```python
from build123d import *

# Parameters (mm, degrees)
SKETCH_R     = 9.65
PAD_DEPTH    = 100
FILLET_R     = 3
POCKET_DEPTH = 3


with BuildPart() as part:
    # Sketch → Pad (new body)
    with BuildSketch(Plane.XY):
        with BuildLine():
            ThreePointArc((0, 12.5), (-12.5, 0), (0, -12.5))
            Line((0, -12.5), (10.5, -12.5))
            Line((10.5, 12.5), (10.5, -12.5))
            Line((0, 12.5), (10.5, 12.5))
        make_face()
        Circle(SKETCH_R, mode=Mode.SUBTRACT)
    extrude(amount=PAD_DEPTH)

    # Fillet
    fillet_edges = [part.edges().sort_by_distance(p)[0] for p in [
        (10.5, -12.5, 50),
        (10.5, 12.5, 50),
    ]]
    fillet(fillet_edges, radius=FILLET_R)

    # Sketch001 (on DatumPlane) → Pocket (cut)
    with BuildSketch(Plane(origin=(-12.5, 0, 100), x_dir=(0, 0, -1), z_dir=(-1, 0, 0))):
        Polygon((12.979274, -3.5), (17.020726, -3.5), (19.041452, 0), (17.020726, 3.5), (12.979274, 3.5), (10.958548, 0), align=None)
        Polygon((87.020726, -3.5), (89.041452, 0), (87.020726, 3.5), (82.979274, 3.5), (80.958548, 0), (82.979274, -3.5), align=None)
    extrude(amount=-POCKET_DEPTH, mode=Mode.SUBTRACT)


solid = part.part
```
Input: part model. Units: mm. Frame: model coordinates. A direction names the side the tool comes from. Coordinates: 2 decimals unless noted, no trailing zeros. Write each loop counter-clockwise with the first axis right and the second up, starting at its lowest first coordinate (ties: lowest second). Pieces come first, ordered by that corner, then holes. Notation, with made-up numbers: (79.25, 16.25) -> (101.25, 16.25) arc R24 ccw to (101.25, 47.25) -> close; hole circle Ø7 at (6.25, 2). An arc over 180 degrees is marked (long way). Answer as a JSON object with one key per item and string values.
1. First-contact query: P1, Ø3, axis at x = -11.5, z = 85, coming from the -Y side; P2, Ø1.2, axis at x = -11.5, z = 15, coming from the +Y side; P3, Ø1, axis at y = 10, z = 29, coming from the -X side. Flat tips, straight axial feed; report the tip coordinate or a pass-through.
Result set:
{"P1": "stops at y = -7.5", "P2": "stops at y = 6.12", "P3": "stops at x = -8.12"}
2. Access query for faces 1 (the face through (-11, -3.5, 85)), 2 (the face through (-5.3, 8.4, 0)). Directions: +Z, -Z, +X, -X, +Y, -Y. A direction counts if a zero-diameter tool reaches every point of the face in a straight line with its end or side. Return the directions, or none.
Result set:
{"face 1": "-X", "face 2": "-Z, +X, -X, +Y, -Y"}
3. Mould query, pull axis Y, two halves, no side actions, for faces 3 (the face through (10.5, 0, 49)), 4 (the face through (-12.497, 0.275, 49.3)), 5 (the face through (-11, -3.5, 15)). Classes: released by +Y, released by -Y, zero draft, split by the parting line, or undercut.
Result set:
{"face 3": "zero draft", "face 4": "split by the parting line", "face 5": "undercut"}
4. Section B-B on x = -5.5. Return the cut outline in (y, z), then the cut area to 3 significant figures.
Result set:
{"outline": "(-11.22, 0) -> (-7.93, 0) -> (-7.93, 100) -> (-11.22, 100) -> close; (7.93, 0) -> (11.22, 0) -> (11.22, 100) -> (7.93, 100) -> close", "area": "659 mm2"}
5. Section C-C on y = 7. Return the cut outline in (x, z), then the cut area to 3 significant figures.
Result set:
{"outline": "(-10.36, 0) -> (-6.64, 0) -> (-6.64, 100) -> (-10.36, 100) -> close; (6.64, 0) -> (10.5, 0) -> (10.5, 100) -> (6.64, 100) -> close", "area": "757 mm2"}
6. Material intervals for line 1 (Y direction, x = 0, z = 40); line 2 (X direction, y = 0, z = 36); line 3 (Y direction, x = 3, z = 55), sorted ascending. Write a range as from..to.
Result set:
{"line 1": "y = -12.5..-9.65, 9.65..12.5", "line 2": "x = -12.5..-9.65, 9.65..10.5", "line 3": "y = -12.5..-9.17, 9.17..12.5"}
7. Section A-A on z = 21.5. Return the cut outline in (x, y).
Result set:
{"outline": "(0, -12.5) -> (7.5, -12.5) arc R3 ccw to (10.5, -9.5) -> (10.5, 9.5) arc R3 ccw to (7.5, 12.5) -> (0, 12.5) arc R12.5 ccw to start; hole circle Ø19.3 at (0, 0)"}
